Here's how the part is built. I have some questions about the finished solid (model axes, mm). A direction names the side the tool comes from. Round coordinates to 2 decimals unless told otherwise and drop trailing zeros. Loops run counter-clockwise (first coordinate to the right, second up) from the corner with the lowest first, then second, coordinate; pieces in that order, holes last. Notation, with made-up numbers: M 67,49.5 L 90,49.5 A14 cw 90,59.5 Z; hole C 81.5,24 d1. An arc over 180 degrees is marked long. Answer as a JSON object with one key per item and string values.
from build123d import *

# Parameters (mm, degrees)
SKETCH1_W           = 1920
SKETCH1_H           = 237
BOSS_EXTRUDE1_DEPTH = 40
SKETCH2_W           = 1920
SKETCH2_H           = 317
BOSS_EXTRUDE2_DEPTH = 80
SKETCH3_W           = 23
SKETCH3_H           = 80
CUT_EXTRUDE2_DEPTH  = 1019.081038032
SKETCH6_W           = 80
SKETCH6_H           = 82
CUT_EXTRUDE3_DEPTH  = 1912.128266234
SKETCH7_W           = 60
SKETCH7_H           = 80
CUT_EXTRUDE4_DEPTH  = 1019.081038032
CUT_EXTRUDE5_DEPTH  = 1674


with BuildPart() as part:
    # Sketch1 → Boss-Extrude1 (new body)
    with BuildSketch(Plane.XY):
        Rectangle(SKETCH1_W, SKETCH1_H)
    extrude(amount=BOSS_EXTRUDE1_DEPTH)

    # Sketch2 → Boss-Extrude2 (add)
    with BuildSketch(Plane.XY.offset(40)):
        with Locations((0, 40)):
            Rectangle(SKETCH2_W, SKETCH2_H)
    extrude(amount=BOSS_EXTRUDE2_DEPTH)

    # Sketch3 → Cut-Extrude2 (cut, through all)
    with BuildSketch(Plane(origin=(0, 198.5, 0), x_dir=(1, 0, 0), z_dir=(0, 1, 0))):
        with Locations((-948.5, -80)):
            Rectangle(SKETCH3_W, SKETCH3_H)
        with Locations((948.5, -80)):
            Rectangle(SKETCH3_W, SKETCH3_H)
    extrude(amount=-CUT_EXTRUDE2_DEPTH, mode=Mode.SUBTRACT)

    # Sketch6 → Cut-Extrude3 (cut, through all)
    with BuildSketch(Plane(origin=(937, 0, 0), x_dir=(0, 0, -1), z_dir=(1, 0, 0))):
        with Locations((-80, -77.5)):
            Rectangle(SKETCH6_W, SKETCH6_H)
    extrude(amount=-CUT_EXTRUDE3_DEPTH, mode=Mode.SUBTRACT)

    # Sketch7 → Cut-Extrude4 (cut, through all)
    with BuildSketch(Plane(origin=(0, 198.5, 0), x_dir=(1, 0, 0), z_dir=(0, 1, 0))):
        with Locations((-907, -80)):
            Rectangle(SKETCH7_W, SKETCH7_H)
        with Locations((907, -80)):
            Rectangle(SKETCH7_W, SKETCH7_H)
    extrude(amount=-CUT_EXTRUDE4_DEPTH, mode=Mode.SUBTRACT)

    # Sketch8 → Cut-Extrude5 (cut)
    with BuildSketch(Plane(origin=(837, 0, 0), x_dir=(0, 0, -1), z_dir=(1, 0, 0))):
        Polygon((-117, 158.5), (-117, 195.5), (-80, 195.5), (-80, 198.5), (-120, 198.5), (-120, 158.5), align=None)
    extrude(amount=-CUT_EXTRUDE5_DEPTH, mode=Mode.SUBTRACT)


solid = part.part
Item 1: I want a section at D-D, the plane z = 21.5. Please give me the cut outline in (x, y).
Resolved:
{"outline": "M -960,-118.5 L 960,-118.5 L 960,118.5 L -960,118.5 Z"}
Item 2: On a 3-axis mill with a long thin cutter (end or side, diameter ignored), from which of +Z, -Z, +X, -X, +Y, -Y can I reach the whole of each face in a straight line? I mean faces 5 (the face through (-13, 118.5, 20)), 6 (the face through (-877, 83, 81)), 7 (the face through (837, 187, 118)), 8 (the face through (12, -36.5, 81)). Say none if no direction works.
Resolved:
{"face 5": "-Z, +X, -X, +Y", "face 6": "+Z, -X, +Y, -Y", "face 7": "+Z, +Y", "face 8": "+Z, +X, -X, -Y"}
Item 3: Please list where these lines run through material, in increasing order: probe 1 along Z at (x, y) = (427, -75.5); probe 2 along Y at (x, z) = (421, 49); probe 3 along Y at (x, z) = (-346, 22.5). Write a range as from..to.
Resolved:
{"probe 1": "0..40", "probe 2": "-36.5..198.5", "probe 3": "-118.5..118.5"}
Item 4: I want a section at B-B, the plane x = -481. Please give me the cut outline in (y, z), then the cut area to 3 significant figures.
Resolved:
{"outline": "M -118.5,0 L 118.5,0 L 118.5,40 L 198.5,40 L 198.5,80 L 195.5,80 L 195.5,117 L 158.5,117 L 158.5,120 L -36.5,120 L -36.5,40 L -118.5,40 Z", "area": "28,000 mm²"}
Item 5: I'm going to push flat-ended pins straight in: pin 1 Ø24 at (x, z) = (163.5, 97.5) entering from -Y; pin 2 Ø3.5 at (x, z) = (318.5, 119) entering from +Y; pin 3 Ø1 at (x, y) = (-18, 148) entering from -Z. Where does each tip first touch, or does it pass through?
Resolved:
{"pin 1": "y = -36.5", "pin 2": "y = 158.5", "pin 3": "z = 40"}
Item 6: I want a section at A-A, the plane z = 100.5. Please give me the cut outline in (x, y), then the cut area to 3 significant figures.
Resolved:
{"outline": "M -877,-36.5 L 877,-36.5 L 877,198.5 L 837,198.5 L 837,195.5 L -837,195.5 L -837,198.5 L -877,198.5 Z", "area": "407,000 mm²"}
Item 7: If we mould it in two halves opening along X, with no side actions, what happens to faces 1 (the face through (-13, -118.5, 20)), 2 (the face through (12, 177, 117)), 3 (the face through (12, 195.5, 99)), 4 (the face through (877, 83, 81))? For each: pulls with the +X half, pulls with the -X half, needs draft (parallel to the pull), parting line crosses it, or undercut.
Resolved:
{"face 1": "needs draft", "face 2": "undercut", "face 3": "undercut", "face 4": "pulls with the +X half"}
Item 8: I want a section at C-C, the plane y = 91. Please give me the cut outline in (x, z).
Resolved:
{"outline": "M -960,0 L 960,0 L 960,40 L 877,40 L 877,120 L -877,120 L -877,40 L -960,40 Z"}
